The listing builds one solid part. Answer for the finished solid, in the listing's coordinates (mm). Face numbers are marked on the shaded views. Coordinates: 2 decimals unless noted, no trailing zeros. Write each loop counter-clockwise with the first axis right and the second up, starting at its lowest first coordinate (ties: lowest second). Pieces come first, ordered by that corner, then holes.
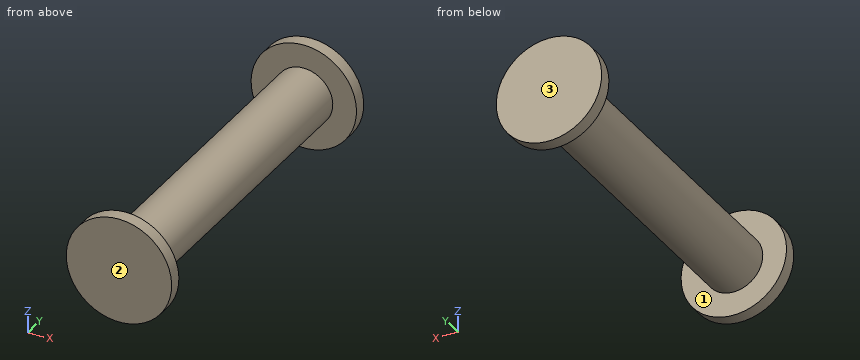
```python
from build123d import *

# Parameters (mm, degrees)
SKETCH1_R           = 2.2
BOSS_EXTRUDE1_DEPTH = 24.5
SKETCH2_R           = 4
BOSS_EXTRUDE2_DEPTH = 1
BOSS_EXTRUDE3_START = 1
SKETCH3_R           = 4
BOSS_EXTRUDE3_DEPTH = 1


with BuildPart() as part:
    # Sketch1 → Boss-Extrude1 (new body)
    with BuildSketch(Plane(origin=(0, 0, 0), x_dir=(1, 0, 0), z_dir=(0, 1, 0))):
        with Locations(Location((0, 0, 0), (0, 0, 270))):
            Circle(SKETCH1_R)
    extrude(amount=BOSS_EXTRUDE1_DEPTH)

    # Sketch2 → Boss-Extrude2 (add)
    with BuildSketch(Plane(origin=(0, 24.5, 0), x_dir=(1, 0, 0), z_dir=(0, 1, 0))):
        with Locations(Location((0, 0, 0), (0, 0, 270))):
            Circle(SKETCH2_R)
    extrude(amount=BOSS_EXTRUDE2_DEPTH)

    # Sketch3 → Boss-Extrude3 (add)
    with BuildSketch(Plane.XZ.offset(BOSS_EXTRUDE3_START)):
        with Locations(Location((0, 0, 0), (0, 0, 90))):
            Circle(SKETCH3_R)
    extrude(amount=-BOSS_EXTRUDE3_DEPTH)


solid = part.part
```
(1) For a pull along Y with two mould halves and no side action, classify the marked faces 1, 2 and 3 as pulls with the +Y half, pulls with the -Y half, needs draft (parallel to the pull), parting line crosses it, or undercut.
(2) Section C-C, the plane z = 0 is taken. Write down the section's boundary in (x, y), plus the area to 3 significant figures.
(3) Section A-A, the plane x = 3.5 is taken. Write down the section's boundary in (y, z), plus the area to 3 significant figures.
(4) Each of these flat-tipped pins is pushed along its axis until it touches: pin 1 (1.5 mm diameter, centred on x = 2, y = 5, fed in from +Z); pin 2 (1 mm diameter, centred on y = 4.5, z = 0, fed in from +X); pin 3 (1 mm diameter, centred on x = 0.5, y = 20.5, fed in from +Z). Where does it stop, or does it pass through?
(5) Find the intervals of material crossed by probe 1 along Y at (x, z) = (1.5, 3.25); probe 2 along Z at (x, y) = (-1.75, 13.75); probe 3 along Z at (x, y) = (2, 5.5), in increasing order.
(6) Section D-D, the plane y = 17 is taken. Write down the section's boundary in (x, z), plus the area to 3 significant figures.
(7) Section B-B, the plane x = 0 is taken. Write down the section's boundary in (y, z).
Solution:
1. face 1: undercut
1. face 2: pulls with the -Y half
1. face 3: pulls with the +Y half
2. outline: (-4, -1) - (4, -1) - (4, 0) - (2.2, 0) - (2.2, 24.5) - (4, 24.5) - (4, 25.5) - (-4, 25.5) - (-4, 24.5) - (-2.2, 24.5) - (-2.2, 0) - (-4, 0) - close
2. area: 124 mm2
3. outline: (-1, -1.94) - (0, -1.94) - (0, 1.94) - (-1, 1.94) - close; (24.5, -1.94) - (25.5, -1.94) - (25.5, 1.94) - (24.5, 1.94) - close
3. area: 7.75 mm2
4. pin 1: stops at z = 1.81
4. pin 2: stops at x = 2.2
4. pin 3: stops at z = 2.2
5. probe 1: y = -1 to 0, 24.5 to 25.5
5. probe 2: z = -1.33 to 1.33
5. probe 3: z = -0.92 to 0.92
6. outline: circle Ø4.4 at (0, 0)
6. area: 15.2 mm2
7. outline: (-1, -4) - (0, -4) - (0, -2.2) - (24.5, -2.2) - (24.5, -4) - (25.5, -4) - (25.5, 4) - (24.5, 4) - (24.5, 2.2) - (0, 2.2) - (0, 4) - (-1, 4) - close
